For this review, use the dimensioned drawing (mm, ordinates from the lowest corner) and the shaded views. Give positions to 0.01 mm unless a question says otherwise; leave off trailing zeros. Write each loop counter-clockwise with the first axis right and the second up, starting at its lowest first coordinate (ties: lowest second). Pieces come first, ordered by that corner, then holes. Notation, with made-up numbers: M -36,27.5 L -14,27.5 A34 cw -14,59.5 Z; hole C -17.5,13 d11. An arc over 180 degrees is marked long. Answer in a Markdown table with one row per item.
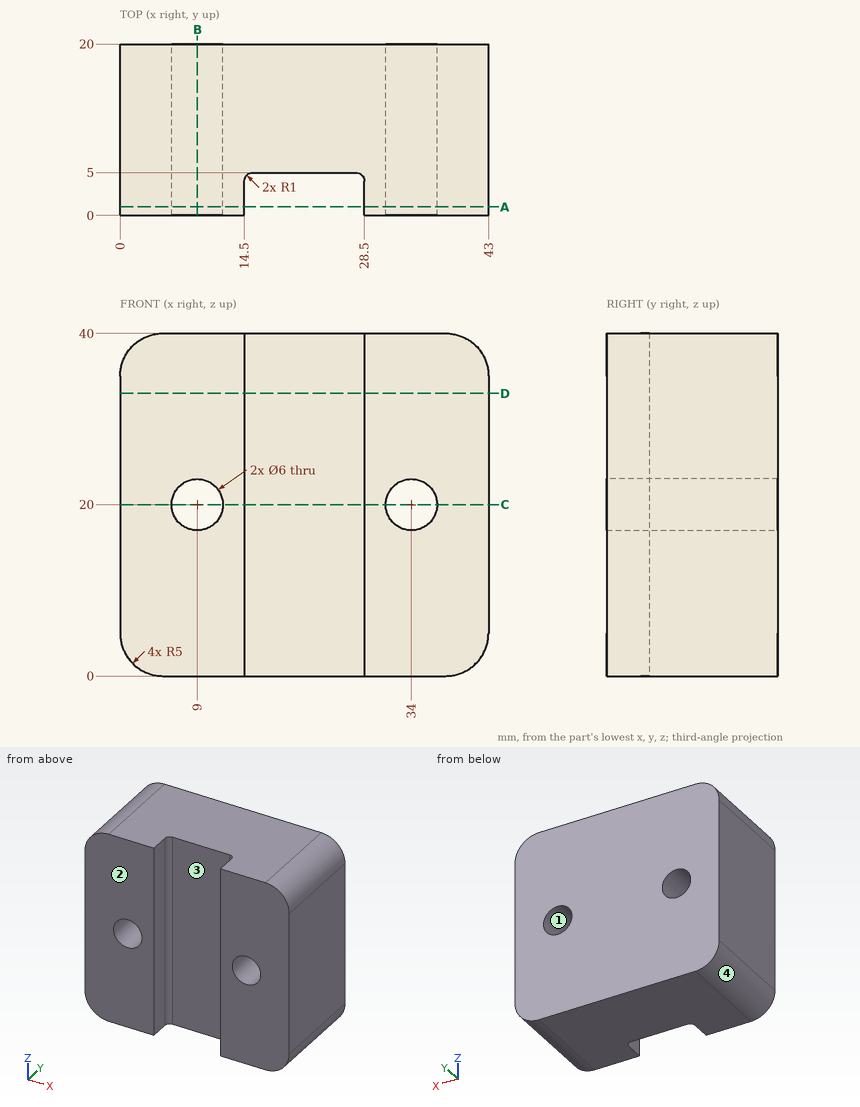
1) To check wall thickness, follow probe 1 along X at (y, z) = (8.75, 20); probe 2 along X at (y, z) = (2.75, 30.5); probe 3 along X at (y, z) = (2.25, 18). State the ranges of each line that lie inside material, in increasing order. Write a range as [from, to].
Geometry says:
| item | result |
|---|---|
| probe 1 | [0, 6], [12, 31], [37, 43] |
| probe 2 | [0, 14.5], [28.5, 43] |
| probe 3 | [0, 6.76], [11.24, 14.5], [28.5, 31.76], [36.24, 43] |
2) Add section A-A (y = 1). Write out the cut boundary in (x, z), and give its area (3 significant figures).
Geometry says:
| item | result |
|---|---|
| outline | M 0,5 A5 ccw 5,0 L 14.5,0 L 14.5,40 L 5,40 A5 ccw 0,35 Z; M 28.5,0 L 38,0 A5 ccw 43,5 L 43,35 A5 ccw 38,40 L 28.5,40 Z; hole C 9,20 d6; hole C 34,20 d6 |
| area | 1,080 mm^2 |
3) Add section C-C (z = 20). Write out the cut boundary in (x, y).
Geometry says:
| item | result |
|---|---|
| outline | M 0,0 L 6,0 L 6,20 L 0,20 Z; M 12,0 L 14.5,0 L 14.5,4 A1 cw 15.5,5 L 27.5,5 A1 cw 28.5,4 L 28.5,0 L 31,0 L 31,20 L 12,20 Z; M 37,0 L 43,0 L 43,20 L 37,20 Z |
4) Add section D-D (z = 33). Write out the cut boundary in (x, y).
Geometry says:
| item | result |
|---|---|
| outline | M 0,0 L 14.5,0 L 14.5,4 A1 cw 15.5,5 L 27.5,5 A1 cw 28.5,4 L 28.5,0 L 43,0 L 43,20 L 0,20 Z |
5) Insertion check: P1, Ø3.5, axis at x = 23, z = 17, coming from the -Y side; P2, Ø5, axis at x = 34, z = 20, coming from the -Y side. Each pin has a flat end and moves straight along its axis. Give the tip position at first contact, or say it passes through.
Geometry says:
| item | result |
|---|---|
| P1 | y = 5 |
| P2 | through |
6) The part is to be moulded in two halves that separate along X. For the marked faces 1, 2, 3 and 4, say which applies: released by +X, released by -X, zero draft, split by the parting line, or undercut.
Geometry says:
| item | result |
|---|---|
| face 1 | undercut |
| face 2 | zero draft |
| face 3 | undercut |
| face 4 | released by -X |
7) Add section B-B (x = 9). Write out the cut boundary in (y, z), and give its area (3 significant figures).
Geometry says:
| item | result |
|---|---|
| outline | M 0,0 L 20,0 L 20,17 L 0,17 Z; M 0,23 L 20,23 L 20,40 L 0,40 Z |
| area | 680 mm^2 |
